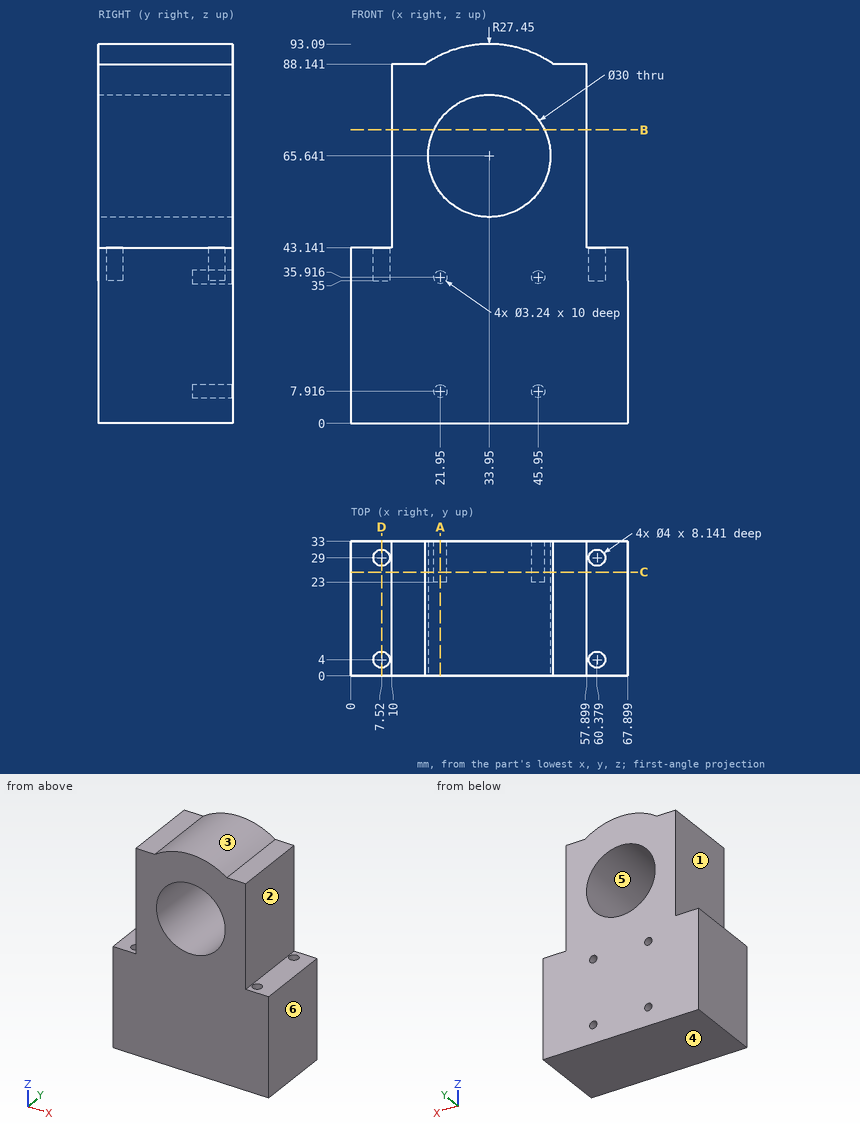
Geometry: see drawing. Coordinates: mm, zero at the bounding-box minimum. A direction names the side the tool comes from. Coordinates: 2 decimals unless noted, no trailing zeros. Loops run counter-clockwise (first coordinate to the right, second up) from the corner with the lowest first, then second, coordinate; pieces in that order, holes last.
Q1. Cut plane B-B (z = 72). Output: boundary loops of the cut face in (x, y) (1 decimal).
Q2. Cut plane D-D (x = 7.52). Output: boundary loops of the cut face in (y, z).
Q3. Set-up query: the marked faces 1, 2 and 3. Return all of +Z, -Z, +X, -X, +Y, -Y with unobstructed straight access to the full face (end or side cutting, diameter ignored); none if empty.
Q4. Cut plane A-A (x = 21.95). Output: boundary loops of the cut face in (y, z) (1 decimal), then the cut area to 3 significant figures.
Q5. Cut plane C-C (y = 25.5). Give the number of separate pieces and of enclosed holes in the cut face, then the cut area to 3 significant figures.
Q6. Material intervals for line 1 (Z direction, x = 21, y = 27) (1 decimal); line 2 (Y direction, x = 7, z = 37); line 3 (Z direction, x = 8, y = 27.5), sorted ascending.
Q7. Draft query along X for the marked faces 4, 5 and 6. Return one class per face: +X half, -X half, draft (parallel to the pull), parting line (faces both ways), or undercut.
Q8. Contact query for flat-ended pins moving along their axis: pin 1 (16.5 mm diameter, centred on y = 15.5, z = 69, fed in from -X); pin 2 (3 mm diameter, centred on x = 59.5, y = 28.5, fed in from +Z); pin 3 (10 mm diameter, centred on y = 12, z = 59.5, fed in from +X). Output: stop coordinate, or through.
Working result:
1. outline: (10, 0) - (20.4, 0) - (20.4, 33) - (10, 33) - close; (47.5, 0) - (57.9, 0) - (57.9, 33) - (47.5, 33) - close
2. outline: (0, 0) - (33, 0) - (33, 43.14) - (31, 43.14) - (31, 35) - (27, 35) - (27, 43.14) - (6, 43.14) - (6, 35) - (2, 35) - (2, 43.14) - (0, 43.14) - close
3. face 1: +Z, -X, +Y, -Y
3. face 2: +Z, +X, +Y, -Y
3. face 3: +Z, +Y, -Y
4. outline: (0, 0) - (33, 0) - (33, 6.3) - (23, 6.3) - (23, 9.5) - (33, 9.5) - (33, 34.3) - (23, 34.3) - (23, 37.5) - (33, 37.5) - (33, 56.6) - (0, 56.6) - close; (0, 74.6) - (33, 74.6) - (33, 90.3) - (0, 90.3) - close
4. area: 2,320 mm2
5. separate pieces: 1
5. enclosed holes: 5
5. area: 4,450 mm2
6. line 1: z = 0 to 6.6, 9.2 to 34.6, 37.2 to 58.1, 73.2 to 89.8
6. line 2: y = 0 to 2.07, 5.93 to 27.07, 30.93 to 33
6. line 3: z = 0 to 35
7. face 4: draft
7. face 5: undercut
7. face 6: +X half
8. pin 1: stops at x = 10
8. pin 2: stops at z = 43.14
8. pin 3: stops at x = 57.9
